Could you check a few things on this model? Use its own coordinates, in mm. Face numbers are marked on the shaded views. A direction names the side the tool comes from. Round coordinates to 2 decimals unless told otherwise and drop trailing zeros. Loops run counter-clockwise (first coordinate to the right, second up) from the corner with the lowest first, then second, coordinate; pieces in that order, holes last. Notation, with made-up numbers: M -26,22.5 L -15,22.5 A16 ccw -15,30.5 Z; hole C 12.25,68.5 d4. An arc over 180 degrees is marked long. One line per item, written item: value. Start each with the question number.
Q1. Which directions (+Z, -Z, +X, -X, +Y, -Y) give clear straight access to the entire face, cutting with the end or side of a thin tool? Please do the marked faces 1, 2 and 3.
Q2. Imagine slicing it at B-B (x = 5.75). Please give me the cut outline in (y, z), then the cut area to 3 significant figures.
Q3. Please list where these lines run through material, in increasing order: line 1 along Y through (x, z) = (7.25, 52.25); line 2 along Y through (x, z) = (4, -31.25); line 3 along Z through (x, y) = (-5.5, 15).
Q4. Imagine slicing it at A-A (z = -31.25). Please give me the cut outline in (x, y), then the cut area to 4 significant figures.
Q5. I'm going to push flat-ended pins straight in: pin 1 Ø14.5 at (y, z) = (10.5, 19) entering from -X; pin 2 Ø2 at (x, y) = (-10.5, 1) entering from +Z; pin 3 Ø4.5 at (y, z) = (12.5, 2.25) entering from -X; pin 4 Ø5.5 at (y, z) = (9, -45.5) entering from -X. Where does each tip first touch, or does it pass through?
Q6. Imagine slicing it at D-D (y = -2.5). Please give me the cut outline in (x, z), then the cut area to 3 significant figures.
Q7. Imagine slicing it at C-C (x = -4). Please give me the cut outline in (y, z).
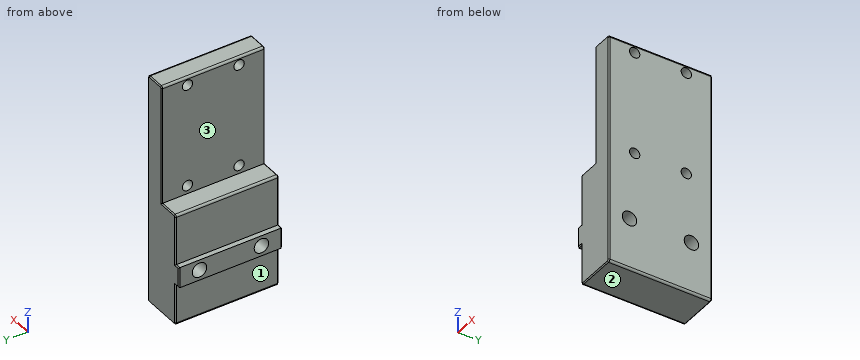
Solid Edge part; units mm, degrees
sketch "Sketch1" plane through (0, 0, 0) normal (0, -1, 0) x (1, 0, 0)
  line L0 (10, 56.25) -> (0, 56.25)
  line L1 (0, 56.25) -> (0, -1.75)
  line L2 (0, -1.75) -> (-10, -1.75)
  line L3 (-10, -1.75) -> (-10, -56.25)
  line L4 (-10, -56.25) -> (10, -56.25)
  line L5 (10, -56.25) -> (10, 56.25)
extrude "Extrusionsausprägung_20" add sketch "Sketch1" along normal mid plane 50
hole "Bohrung_4" at (10, -12.5, 52.25) direction (-1, 0, 0) diameter 5 end up to next
hole "Hole1" at (10, 12.5, 52.25) direction (-1, 0, 0) diameter 5 end up to next
hole "Hole2" at (10, 12.5, 2.25) direction (-1, 0, 0) diameter 5 end up to next
hole "Hole3" at (10, -12.5, 2.25) direction (-1, 0, 0) diameter 5 end up to next
sketch "Sketch2" plane through (0, -25, 0) normal (0, -1, 0) x (0, 0, -1)
  line L0 (26.25, -12.5) -> (36.25, -12.5)
  line L1 (36.25, -12.5) -> (36.25, -10)
  line L2 (36.25, -10) -> (26.25, -10)
  line L3 (26.25, -10) -> (26.25, -12.5)
extrude "Protrusion1" add sketch "Sketch2" against normal up to vertex (50 mm away)
hole "Bohrung_8" at (-12.5, -15, -31.25) direction (1, 0, 0) diameter 7 end up to next
hole "Hole4" at (-12.5, 15, -31.25) direction (1, 0, 0) diameter 7 end up to next
fillet "Verrundung_15" radius 1 5 edges at (-10, 0, -56.25) (10, 0, -56.25) (10, 0, 56.25) (0, 0, 56.25) (-10, 0, -1.75)
chamfer "Fase_9" distance 0.5 angle 45 30 edges at (-4.5, -25, -1.75) (-9.7071, -25, -2.0429) (-10, -25, -14.5) (-11.25, -25, -26.25) (-12.5, -25, -31.25) (-11.25, -25, -36.25) (-10, -25, -45.75) (-9.7071, -25, -55.9571) (0, -25, -56.25) (9.7071, -25, -55.9571) (10, -25, 0) (9.7071, -25, 55.9571) (5, -25, 56.25) (0.2929, -25, 55.9571) (0, -25, 26.75) (-10, 25, -14.5) (-9.7071, 25, -2.0429) (-4.5, 25, -1.75) (0, 25, 26.75) (0.2929, 25, 55.9571) (5, 25, 56.25) (9.7071, 25, 55.9571) (10, 25, 0) (9.7071, 25, -55.9571) (0, 25, -56.25) (-9.7071, 25, -55.9571) (-10, 25, -45.75) (-11.25, 25, -36.25) (-12.5, 25, -31.25) (-11.25, 25, -26.25)
Report:
1. face 1: -Z, -X, +Y, -Y
1. face 2: -Z, +X, -X, +Y, -Y
1. face 3: +Z, -X, +Y, -Y
2. outline: M -25,-55.75 L -24.5,-56.25 L 24.5,-56.25 L 25,-55.75 L 25,55.75 L 24.5,56.25 L -24.5,56.25 L -25,55.75 Z; hole C -15,-31.25 d7; hole C -12.5,2.25 d5; hole C -12.5,52.25 d5; hole C 12.5,2.25 d5; hole C 12.5,52.25 d5; hole C 15,-31.25 d7
2. area: 5,470 mm²
3. line 1: y = -25 to -15, -10 to 10, 15 to 25
3. line 2: y = -25 to -18.5, -11.5 to 11.5, 18.5 to 25
3. line 3: z = -56.25 to -34.75, -27.75 to -1.75
4. outline: M -12.5,-24.5 L -12,-25 L 9.5,-25 L 10,-24.5 L 10,-18.5 L -12.5,-18.5 Z; M -12.5,-11.5 L 10,-11.5 L 10,11.5 L -12.5,11.5 Z; M -12.5,18.5 L 10,18.5 L 10,24.5 L 9.5,25 L -12,25 L -12.5,24.5 Z
4. area: 809.5 mm²
5. pin 1: stops at x = 0
5. pin 2: stops at z = -1.88
5. pin 3: passes through
5. pin 4: stops at x = -10
6. outline: M -12.5,-36.25 L -10,-36.25 L -10,-55.25 A1 ccw -9,-56.25 L 9,-56.25 A1 ccw 10,-55.25 L 10,55.25 A1 ccw 9,56.25 L 1,56.25 A1 ccw 0,55.25 L 0,-1.75 L -9,-1.75 A1 ccw -10,-2.75 L -10,-26.25 L -12.5,-26.25 Z
6. area: 1,690 mm²
7. outline: M -25,-55.75 L -24.5,-56.25 L 24.5,-56.25 L 25,-55.75 L 25,-2.25 L 24.5,-1.75 L -24.5,-1.75 L -25,-2.25 Z; hole C -15,-31.25 d7; hole C 15,-31.25 d7
